from build123d import *

# Parameters (mm, degrees)
FUROS_GUIA_COM_6_0MM1_D       = 6
FUROS_GUIA_COM_6_0MM2_REACH   = 46.246
FUROS_GUIA_COM_6_0MM2_BORE_R  = 3
RESSALTO_EXTRUS_O1_REACH      = 60.94
RESSALTO_EXTRUS_O1_END_RADIUS = 17.5
RESSALTO_EXTRUS_O1_START      = -30
ESBO_O4_R                     = 4
ESBO_O4_R_2                   = 3
RESSALTO_EXTRUS_O2_OUTLINE_W  = 1
RESSALTO_EXTRUS_O2_OUTLINE_H  = 12.963481803


# Read off the part's stored shape, not the designer's step: Ressalto-extrusão2
with BuildPart() as part:
    # Esboço1 → Revolução1 (revolve)
    with BuildSketch(Plane.XY, mode=Mode.PRIVATE) as revolu_o1_sk:
        Polygon((0, -15), (17.5, -15), (17.5, 8), (15, 8), (15, -9), (5, -9), (5, -11.5), (3.25, -11.5), (3.25, -12.5), (0, -12.5), align=None)
    revolve(revolu_o1_sk.sketch.rotate(Axis((0, 0, 0), (0, 1, 0)), 90), axis=Axis((0, 0, 0), (0, 1, 0)))

    # Furos-guia com Ø6.0mm1 (through all)
    with Locations(Plane(origin=(-17.5, 0, 0), x_dir=(0, 0, -1), z_dir=(-1, 0, 0))):
        with Locations((0, 0)):
            Hole(FUROS_GUIA_COM_6_0MM1_D / 2)

    # Furos-guia com Ø6.0mm2 bore (on position points) → Furos-guia com Ø6.0mm2 (cut, up to next)
    with BuildSketch(Plane(origin=(-15.860386273, 0, -7.39581958), x_dir=(0.422618261741, 0, -0.906307787037), z_dir=(-0.906307787037, 0, -0.422618261741)), mode=Mode.PRIVATE) as furos_guia_com_6_0mm2_sk1:
        Circle(FUROS_GUIA_COM_6_0MM2_BORE_R)
    furos_guia_com_6_0mm2_tool1 = extrude(furos_guia_com_6_0mm2_sk1.sketch, amount=-FUROS_GUIA_COM_6_0MM2_REACH, mode=Mode.PRIVATE) & part.part
    add(furos_guia_com_6_0mm2_tool1.solids().sort_by_distance((-15.860386, 0, -7.39582))[0], mode=Mode.SUBTRACT)

    # Ressalto-extrusão1: up to this cylinder (the profile starts outside it)
    ressalto_extrus_o1_end = Plane(origin=(0, 0, 0), z_dir=(0, -1, 0)) * Cylinder(RESSALTO_EXTRUS_O1_END_RADIUS, 157.88, mode=Mode.PRIVATE)
    # Esboço4 → Ressalto-extrusão1 (add, up to the surface)
    with BuildSketch(Plane(origin=(0, 0, 0), x_dir=(0, 0, -1), z_dir=(1, 0, 0)).offset(RESSALTO_EXTRUS_O1_START), mode=Mode.PRIVATE) as ressalto_extrus_o1_sk1:
        with Locations(Location((0, 0, 0), (0, 0, 180))):
            Circle(ESBO_O4_R)
        with Locations(Location((0, 0, 0), (0, 0, 180))):
            Circle(ESBO_O4_R_2, mode=Mode.SUBTRACT)
    ressalto_extrus_o1_tool1 = extrude(ressalto_extrus_o1_sk1.sketch, amount=RESSALTO_EXTRUS_O1_REACH, mode=Mode.PRIVATE) - ressalto_extrus_o1_end
    ressalto_extrus_o1 = ressalto_extrus_o1_tool1.solids().sort_by_distance((-30, 0, -3.886863))[0]
    add(ressalto_extrus_o1)

    # Espelhar3: Ressalto-extrusão1 across plane
    add(ressalto_extrus_o1.mirror(Plane(origin=(0, 0, 0), x_dir=(0, 0, 1), z_dir=(1, 0, 0))))

    # Ressalto-extrusão2 outline → Ressalto-extrusão2 (revolve)
    with BuildSketch(Plane(origin=(0, 0, 0), x_dir=(0, 1, 0), z_dir=(0.4226182617407003, 0, -0.9063077870366496))):
        with Locations((3.5, -23.518259099)):
            Rectangle(RESSALTO_EXTRUS_O2_OUTLINE_W, RESSALTO_EXTRUS_O2_OUTLINE_H)
    revolve(axis=Axis((0, 0, 0), (0.9063077870366496, 0, 0.4226182617407003)))


solid = part.part
Could you check a few things on this model? Use its own coordinates, in mm. A direction names the side the tool comes from. Coordinates: 2 decimals unless noted, no trailing zeros. Order: outer loops, then holes, each group sorted by start corner. A loop starts at its lowest first (then second) coordinate and runs counter-clockwise, first axis right, second up. Notation, with made-up numbers: (28.5, -36) -> (32.5, -36) arc R16 cw to (32.5, -28) -> close; hole circle Ø5 at (83, -34). An arc over 180 degrees is marked (long way). One line per question, with ' | ' between items.
Q1. Imagine slicing it at C-C on x = 0. Please give me the cut outline in (y, z).
Return value:
outline: (-15, -17.5) -> (8, -17.5) -> (8, -15) -> (-9, -15) -> (-9, -5) -> (-11.5, -5) -> (-11.5, -3.25) -> (-12.5, -3.25) -> (-12.5, 3.25) -> (-11.5, 3.25) -> (-11.5, 5) -> (-9, 5) -> (-9, 15) -> (8, 15) -> (8, 17.5) -> (-15, 17.5) -> close
Q2. Thinking about a two-plate mould opening in X: for faces 1 (the face through (23.609, 3.905, -0.867)), 2 (the face through (-30, -3, 1)), 3 (the face through (14.643, -0.619, 3.252)), which applies, pulls with the +X half, pulls with the -X half, needs draft (parallel to the pull), parting line crosses it, or undercut?
Return value:
face 1: needs draft | face 2: pulls with the -X half | face 3: undercut
Q3. Imagine slicing it at D-D on y = 5. Please give me the cut outline in (x, z).
Return value:
outline: circle Ø35 at (0, 0); hole circle Ø30 at (0, 0)
Q4. I'm going to push flat-ended pins straight in: P1, Ø1.5, axis at x = 10.5, y = -8, coming from the -Z side; P2, Ø5, axis at y = 0, z = 0, coming from the -X side (3 decimals); P3, Ø2, axis at x = -1, z = -1.5, coming from the +Y side; P4, Ø11, axis at x = 2, z = 0.5, coming from the +Y side. Where does each tip first touch, or does it pass through?
Return value:
P1: z = -14.53 | P2: through | P3: y = -12.5 | P4: y = -9
Q5. On a 3-axis mill with a long thin cutter (end or side, diameter ignored), from which of +Z, -Z, +X, -X, +Y, -Y can I reach the whole of each face in a straight line? I mean faces 4 (the face through (-8, 8, -13)), 5 (the face through (1.978, -12.007, 2.579)), 6 (the face through (-23.609, 1.532, 3.695)). Say none if no direction works.
Return value:
face 4: +Z, -Z, +X, -X, +Y | face 5: +Y | face 6: -X
Q6. Imagine slicing it at A-A on z = 0. State how many separate pieces and enclosed holes the cut face has, and give its area (4 significant figures).
Return value:
separate pieces: 3 | enclosed holes: 0 | area: 283.5 mm²
Q7. If I drill on L1, parallel to Y at x = 16, z = 0; L2, parallel to X at y = -11.85, z = 0; L3, parallel to Y at x = -21, z = 0, over which ranges is the centre line in solid material (lowest first)?
Return value:
L1: -15 to -3, 3 to 8 | L2: -17.5 to -3.25, 3.25 to 17.5 | L3: -4 to -3, 3 to 4
Q8. Imagine slicing it at B-B on y = 0. Please give me the cut outline in (x, z).
Return value:
outline: (-30, -4) -> (-18.04, -4) -> (-28.88, -9.05) -> (-28.46, -9.96) -> (-14.59, -3.49) arc R15 cw to (-14.7, -3) -> (-30, -3) -> close; (-30, 3) -> (-14.7, 3) arc R15 cw to (14.7, 3) -> (30, 3) -> (30, 4) -> (17.04, 4) arc R17.5 ccw to (-17.04, 4) -> (-30, 4) -> close; (-25.92, -15.4) -> (-25.5, -16.3) -> (-13.75, -10.83) arc R17.5 ccw to (17.04, -4) -> (30, -4) -> (30, -3) -> (14.7, -3) arc R15 cw to (-12.05, -8.93) -> close
